```python
from build123d import *

# Parameters (mm, degrees)
F2_SIZE2 = 2
F2_SIZE  = 2
F3_R     = 2


with BuildPart() as f1:
    # F0 (on Right) → F1 (revolve)
    with BuildSketch(Plane.YZ):
        Polygon((5, 75), (0, 75), (0, 65), (10, 65), (10, 32), (0, 32), (0, 25), (40.8, 20.711747), (40.8, 27), (33.3, 27), (33.3, 65), (40.8, 65), (40.8, 75), (36, 75), (36, 70), (33, 70), (33, 75), (23, 75), (23, 70), (18, 70), (18, 75), (10, 75), (10, 70), (5, 70), align=None)
    revolve(axis=Axis((0, 18.302675, 0), (0, 1, 0)))

    # F2
    f2_edges = [f1.edges().sort_by_distance(p)[0] for p in [
        (0, 40.8, -75),
        (0, 0, -75),
    ]]
    chamfer(f2_edges, length=F2_SIZE, length2=F2_SIZE2)

    # F3
    f3_edges = [f1.edges().sort_by_distance(p)[0] for p in [
        (0, 10, -65),
        (0, 33.3, -65),
        (0, 33.3, -27),
        (0, 10, -32),
    ]]
    fillet(f3_edges, radius=F3_R)


solid = f1.part
```
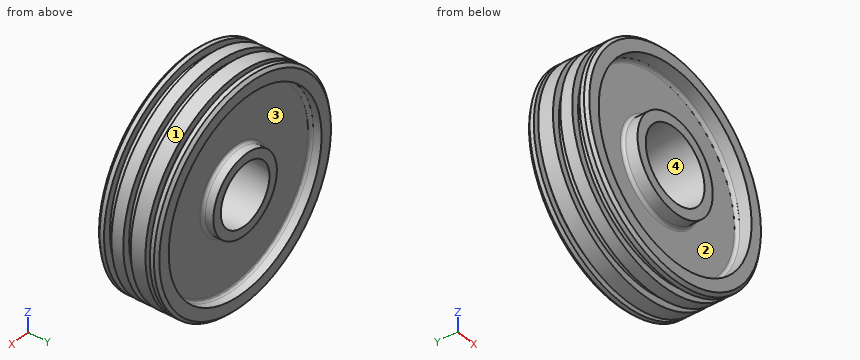
Build history of the part. All positions in model axes, mm. Face numbers are marked on the shaded views. A direction names the side the tool comes from. Round coordinates to 2 decimals unless told otherwise and drop trailing zeros. Write each loop counter-clockwise with the first axis right and the second up, starting at its lowest first coordinate (ties: lowest second). Pieces come first, ordered by that corner, then holes. Notation, with made-up numbers: (-36.75, 72) -> (-19.75, 72) arc R18 cw to (-19.75, 100) -> close; hole circle Ø5 at (-15.75, 72). An arc over 180 degrees is marked (long way). Put each result on its own line as item: value.
Item 1: Tool access for the marked faces 3 and 4: list every direction of +Z, -Z, +X, -X, +Y, -Y with a clear straight run to the whole face (end or side of a thin tool).
Here are the results:
face 3: +Y
face 4: -Y
Item 2: Flat gauge pins, fed straight in: P1, Ø4, axis at x = -58.5, y = 5, coming from the +Z side; P2, Ø1, axis at y = 7, z = 1, coming from the +X side; P3, Ø4, axis at x = -41.5, z = 4, coming from the +Y side. Where does each tip first touch, or does it go through?
Here are the results:
P1: stops at z = 49.32
P2: stops at x = 70
P3: stops at y = 33.3
Item 3: Slice it at A-A, the plane y = 15. Give the cut face in (x, z).
Here are the results:
outline: circle Ø150 at (0, 0); hole circle Ø46.85 at (0, 0)
Item 4: Two-plate mould, pull along X, no slides. Class the marked faces 1 and 2: pulls with the +X half, pulls with the -X half, needs draft (parallel to the pull), parting line crosses it, or undercut.
Here are the results:
face 1: parting line crosses it
face 2: undercut
Item 5: Wall check: probe 1 along Y at (x, z) = (54.5, -50.5); probe 2 along X at (y, z) = (37, 0); probe 3 along Y at (x, z) = (-29.5, -45.5). Give the ranges that are in metal, low to high. Write a range as from..to.
Here are the results:
probe 1: y = 1.3..5, 10..18, 23..33, 36..39.5
probe 2: x = -75..-65, -27..-21.11, 21.11..27, 65..75
probe 3: y = 10..33.3
